Model file for the job. Use its own axes, mm. Coordinates: 2 decimals unless noted, no trailing zeros. Order: outer loops, then holes, each group sorted by start corner. A loop starts at its lowest first (then second) coordinate and runs counter-clockwise, first axis right, second up.
from build123d import *

# Parameters (mm, degrees)
EXTRUDE_1_DEPTH = 20
FILLET_1_R      = 2


with BuildPart() as part:
    # 草图1 → 凸台-拉伸1 (new body)
    with BuildSketch(Plane(origin=(0, 0, 0), x_dir=(0, 0, -1), z_dir=(1, 0, 0))):
        Polygon((0, 25.980762114), (0, 0), (15, 0), align=None)
        Polygon((0, 25.980762114), (-15, 0), (0, 0), align=None)
    extrude(amount=EXTRUDE_1_DEPTH)

    # 圆角1
    fillet_1_edges = [part.edges().sort_by_distance(p)[0] for p in [
        (10, 0, -15),
        (10, 0, 15),
        (10, 25.980762114, 0),
    ]]
    fillet(fillet_1_edges, radius=FILLET_1_R)


solid = part.part
Q1. Probe line 1 (Y direction, x = 14, z = 4); line 2 (Y direction, x = 14, z = -8.25); line 3 (Z direction, x = 15, y = 1.5). List the from-to ranges inside material, lowest first.
Established:
line 1: y = 0 to 19.05
line 2: y = 0 to 11.69
line 3: z = -13.47 to 13.47
Q2. Cut at A-A, the plane x = 6.5. List the corners of the cut face in (y, z).
Established:
outline: (0, -11.54) arc R2 ccw to (3, -13.27) - (22.98, -1.73) arc R2 ccw to (22.98, 1.73) - (3, 13.27) arc R2 ccw to (0, 11.54) - close
Q3. Cut at B-B, the plane y = 18.75. List the corners of the cut face in (x, z), plus the area to 3 significant figures.
Established:
outline: (0, -4.17) - (20, -4.17) - (20, 4.17) - (0, 4.17) - close
area: 167 mm2
Q4. Drop flat-ended pins along their axis: P1, Ø10, axis at x = 17.5, y = 21, coming from the -Z side; P2, Ø8, axis at x = 17.5, y = 19, coming from the -Z side; P3, Ø2, axis at x = 7.5, y = 8, coming from the -Z side. Give the stop position or say it passes through.
Established:
P1: stops at z = -5.76
P2: stops at z = -6.34
P3: stops at z = -10.96
Q5. Cut at C-C, the plane z = -4.25. List the corners of the cut face in (x, y).
Established:
outline: (0, 0) - (20, 0) - (20, 18.62) - (0, 18.62) - close
